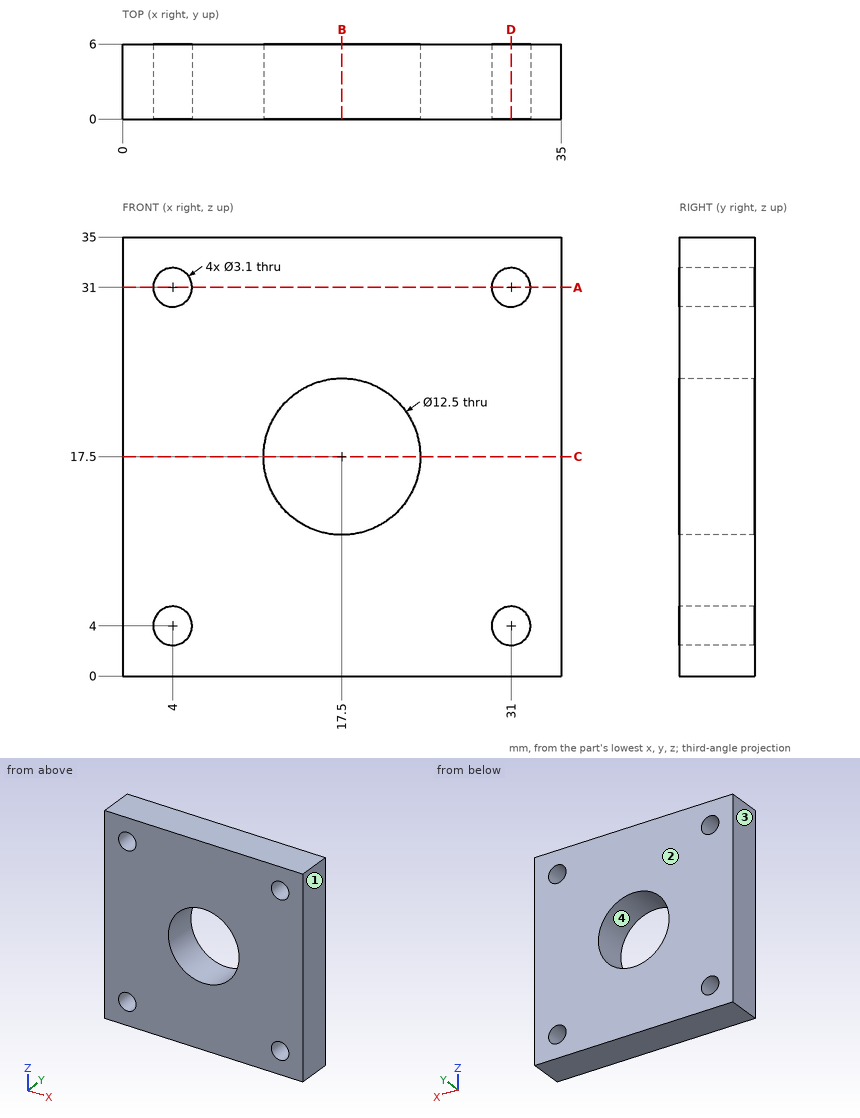
Check sheet for the drawn part. Datum: minimum x, y, z corner. Units: mm. Round coordinates to 2 decimals unless told otherwise and drop trailing zeros. Order: outer loops, then holes, each group sorted by start corner. A loop starts at its lowest first (then second) coordinate and runs counter-clockwise, first axis right, second up. Notation, with made-up numbers: (46.25, -9) -> (83.25, -9) arc R19 ccw to (83.25, 6) -> close; hole circle Ø7 at (62.5, 33.5). An arc over 180 degrees is marked (long way). Use CSV: the item, a comma, the result in double quotes.
(1) Cross-section at D-D (x = 31). Record the boundary of the cut face in (y, z).
Worked out:
outline,"(0, 0) -> (6, 0) -> (6, 2.45) -> (0, 2.45) -> close; (0, 5.55) -> (6, 5.55) -> (6, 29.45) -> (0, 29.45) -> close; (0, 32.55) -> (6, 32.55) -> (6, 35) -> (0, 35) -> close"
(2) Cross-section at A-A (z = 31). Record the boundary of the cut face in (x, y).
Worked out:
outline,"(0, 0) -> (2.45, 0) -> (2.45, 6) -> (0, 6) -> close; (5.55, 0) -> (29.45, 0) -> (29.45, 6) -> (5.55, 6) -> close; (32.55, 0) -> (35, 0) -> (35, 6) -> (32.55, 6) -> close"
(3) Draft check along X on the marked faces 1, 2, 3 and 4. Enter one of: pulls with the +X half, pulls with the -X half, needs draft (parallel to the pull), parting line crosses it, or undercut.
Worked out:
face 1,"pulls with the +X half"
face 2,"needs draft"
face 3,"pulls with the -X half"
face 4,"undercut"
(4) Depth check by flat-ended pin: pin 1 (4 mm diameter, centred on x = 4, z = 4, fed in from +Y). Enter the tip coordinate at first touch or a pass-through.
Worked out:
pin 1,"y = 6"
(5) Material ranges on line 1 along X through (y, z) = (2.4, 4); line 2 along X through (y, z) = (1.95, 17.5), recorded low to high. Write a range as from..to.
Worked out:
line 1,"0..2.45, 5.55..29.45, 32.55..35"
line 2,"0..11.25, 23.75..35"
(6) Cross-section at C-C (z = 17.5). Record the boundary of the cut face in (x, y).
Worked out:
outline,"(0, 0) -> (11.25, 0) -> (11.25, 6) -> (0, 6) -> close; (23.75, 0) -> (35, 0) -> (35, 6) -> (23.75, 6) -> close"
(7) Cross-section at B-B (x = 17.5). Record the boundary of the cut face in (y, z).
Worked out:
outline,"(0, 0) -> (6, 0) -> (6, 11.25) -> (0, 11.25) -> close; (0, 23.75) -> (6, 23.75) -> (6, 35) -> (0, 35) -> close"
